from build123d import *

# Parameters (mm, degrees)
F0_W     = 0.8
F0_H     = 0.8
F0_H_2   = 11.4
F0_W_2   = 7.8
F1_DEPTH = 20
F2_W     = 13.8
F2_H     = 17.4
F2_W_2   = 9.4
F2_H_2   = 13
F2_W_3   = 7.8
F2_H_3   = 11.4
F3_DEPTH = 2


with BuildPart() as f1:
    # F0 (on Top) → F1 (new body)
    with BuildSketch(Plane.XY):
        with Locations((0.4, -0.4)):
            Rectangle(F0_W, F0_H)
        with Locations((0.4, -6.5)):
            Rectangle(F0_W, F0_H_2)
        with Locations((0.4, -12.6)):
            Rectangle(F0_W, F0_H)
        with Locations((4.7, -12.6)):
            Rectangle(F0_W_2, F0_H)
        with Locations((4.7, -0.4)):
            Rectangle(F0_W_2, F0_H)
        with Locations((9, -0.4)):
            Rectangle(F0_W, F0_H)
        with Locations((9, -6.5)):
            Rectangle(F0_W, F0_H_2)
        with Locations((9, -12.6)):
            Rectangle(F0_W, F0_H)
    extrude(amount=F1_DEPTH)

    # F2 (on face) → F3 (join)
    with BuildSketch(Plane.XY.offset(20)):
        with Locations((4.7, -6.5)):
            Rectangle(F2_W, F2_H)
        with Locations((4.7, -6.5)):
            Rectangle(F2_W_2, F2_H_2, mode=Mode.SUBTRACT)
        with Locations((4.7, -6.5)):
            Rectangle(F2_W_2, F2_H_2)
        with Locations((4.7, -6.5)):
            Rectangle(F2_W_3, F2_H_3, mode=Mode.SUBTRACT)
    extrude(amount=F3_DEPTH)


solid = f1.part
CAD build for the part. Positions are in the model's coordinates, mm. A direction names the side the tool comes from. Coordinates: 2 decimals unless noted, no trailing zeros. Loops run counter-clockwise (first coordinate to the right, second up) from the corner with the lowest first, then second, coordinate; pieces in that order, holes last. Notation, with made-up numbers: (76, 61) -> (130, 61) arc R38 cw to (130, 99) -> close; hole circle Ø4 at (57.25, 19). An arc over 180 degrees is marked (long way). One line per item, written item: value.
1. Slice it at C-C on z = 17.5. Write the cut outline in (x, y).
Answers:
outline: (0, -13) -> (9.4, -13) -> (9.4, 0) -> (0, 0) -> close; hole (0.8, -12.2) -> (8.6, -12.2) -> (8.6, -0.8) -> (0.8, -0.8) -> close
2. Which spindle directions (+Z, -Z, +X, -X, +Y, -Y) get a long thin tool onto all of the face, cutting with end or side? Do faces 1 (the face through (9.4, -7, 10)), 2 (the face through (11.6, -7, 21)), 3 (the face through (5, -12.2, 11)), 4 (the face through (0, -6, 10)), 5 (the face through (5, 0, 10)). Say none if no direction does.
Answers:
face 1: -Z, +X, +Y, -Y
face 2: +Z, -Z, +X, +Y, -Y
face 3: +Z, -Z
face 4: -Z, -X, +Y, -Y
face 5: -Z, +X, -X, +Y
3. Flat gauge pins, fed straight in: P1, Ø4.5, axis at x = 3.5, z = 14, coming from the -Y side; P2, Ø7, axis at x = 3.5, y = -7.5, coming from the -Z side; P3, Ø9, axis at y = -7.5, z = 8.5, coming from the -X side; P4, Ø1, axis at x = 5, z = 6.5, coming from the +Y side. Where does each tip first touch, or does it go through?
Answers:
P1: stops at y = -13
P2: stops at z = 0
P3: stops at x = 0
P4: stops at y = 0
4. Slice it at D-D on y = -0.5. Write the cut outline in (x, z), and give its area (3 significant figures).
Answers:
outline: (-2.2, 20) -> (0, 20) -> (0, 0) -> (9.4, 0) -> (9.4, 20) -> (11.6, 20) -> (11.6, 22) -> (-2.2, 22) -> close
area: 216 mm^2
5. Drill centre lines: line 1 (Y direction, x = 5.5, z = 5); line 2 (X direction, y = -5.75, z = 15); line 3 (X direction, y = -11, z = 20.5). Where is each one in solid material? Low to high. Write a range as [from, to].
Answers:
line 1: y = [-13, -12.2], [-0.8, 0]
line 2: x = [0, 0.8], [8.6, 9.4]
line 3: x = [-2.2, 0.8], [8.6, 11.6]
6. Slice it at A-A on x = 3.5. Write the cut outline in (y, z), and give its area (3 significant figures).
Answers:
outline: (-15.2, 20) -> (-13, 20) -> (-13, 0) -> (-12.2, 0) -> (-12.2, 22) -> (-15.2, 22) -> close; (-0.8, 0) -> (0, 0) -> (0, 20) -> (2.2, 20) -> (2.2, 22) -> (-0.8, 22) -> close
area: 44.0 mm^2
7. Slice it at B-B on y = -4.5. Write the cut outline in (x, z), and give its area (3 significant figures).
Answers:
outline: (-2.2, 20) -> (0, 20) -> (0, 0) -> (0.8, 0) -> (0.8, 22) -> (-2.2, 22) -> close; (8.6, 0) -> (9.4, 0) -> (9.4, 20) -> (11.6, 20) -> (11.6, 22) -> (8.6, 22) -> close
area: 44.0 mm^2
8. Pull direction Y, two halves, no side cores. Call faces 6 (the face through (5, -13, 10)), 7 (the face through (11, -6, 20)), 8 (the face through (5, -0.8, 11)), 9 (the face through (8.6, -7, 11)): pulls with the +Y half, pulls with the -Y half, needs draft (parallel to the pull), parting line crosses it, or undercut.
Answers:
face 6: pulls with the -Y half
face 7: needs draft
face 8: undercut
face 9: undercut
